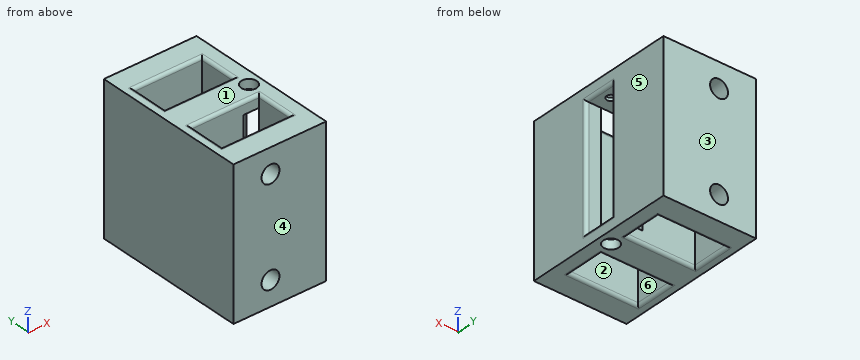
Autodesk Inventor part; units mm, degrees
ref_plane "YZ Plane" through (0, 0, 0) normal (1, 0, 0) x (0, 1, 0)
ref_plane "XZ Plane" through (0, 0, 0) normal (0, 1, 0) x (-1, 0, 0)
ref_plane "XY Plane" through (0, 0, 0) normal (0, 0, 1) x (1, 0, 0)
sketch "スケッチ1" plane through (0, 0, 0) normal (0, 1, 0) x (-1, 0, 0)
  line L0 (0, 0) -> (-30, 0)
  line L1 (-30, 0) -> (-30, -47.5)
  line L2 (-30, -47.5) -> (0, -47.5)
  line L3 (0, -47.5) -> (0, 0)
  dimension "d0" = 30
  dimension "d1" = 47.5
extrude "押し出し1" add sketch "スケッチ1" along normal blind 50
ref_plane "作業平面1" through (30, 0, 0) normal (1, 0, 0) x (0, 0, -1)
sketch "スケッチ2" plane through (30, 0, 0) normal (1, 0, 0) x (0, 0, -1)
  line L0 (4, 30) -> (43.5, 30)
  line L1 (43.5, 30) -> (43.5, 20)
  line L2 (43.5, 20) -> (4, 20)
  line L3 (4, 20) -> (4, 30)
  line L4 (0, 0) -> (0, 50)
  line L5 (0, 0) -> (0, 50)
  line L6 (0, 50) -> (47.5, 50)
  point P0 (0, 25)
  point P1 (4, 25)
  point P2 (0, 25)
  point P3 (23.75, 30)
  point P4 (23.75, 50)
  point P5 (23.75, 50)
  dimension "d5" = 39.5
  dimension "d6" = 10
  dimension "d7" = 0
  dimension "d8" = 0
extrude "押し出し2" cut sketch "スケッチ2" against normal blind 10
sketch "スケッチ3" plane through (0, 0, 0) normal (0, 0, 1) x (1, 0, 0)
  line L0 (3, 42) -> (25, 42)
  line L1 (25, 42) -> (25, 30)
  line L2 (25, 30) -> (3, 30)
  line L3 (3, 30) -> (3, 42)
  line L4 (0, 50) -> (30, 50)
  line L5 (3, 20) -> (25, 20)
  line L6 (25, 20) -> (25, 8)
  line L7 (25, 8) -> (3, 8)
  line L8 (3, 8) -> (3, 20)
  line L9 (0, 0) -> (30, 0)
  line L10 (0, 0) -> (0, 50)
  point P0 (14, 42)
  point P1 (15, 50)
  point P2 (15, 50)
  point P3 (14, 8)
  point P4 (15, 0)
  point P5 (15, 0)
  dimension "d11" = 22
  dimension "d12" = 12
  dimension "d13" = 8
  dimension "d14" = 22
  dimension "d15" = 12
  dimension "d16" = 8
  dimension "d48" = 3
  dimension "d49" = 3
extrude "押し出し3" cut sketch "スケッチ3" against normal through all
ref_plane "作業平面2" through (0, 50, 0) normal (0, 1, 0) x (1, 0, 0)
sketch "スケッチ4" plane through (0, 50, 0) normal (0, 1, 0) x (1, 0, 0)
  line L0 (30, 57) -> (30, -9.5)
  line L1 (30, 47.5) -> (0, 47.5)
  line L2 (0, 0) -> (30, 0)
  line L3 (0, 47.5) -> (0, 0)
  point P0 (12, 39.5)
  point P1 (12, 8)
  dimension "d24" = 8
  dimension "d25" = 8
  dimension "d52" = 12
  dimension "d53" = 12
hole "穴1" at (12, 50, -39.5) at (12, 50, -8) direction (0, -1, 0) diameter 5.8 depth 7
sketch "スケッチ5" plane through (0, 0, 0) normal (0, 0, 1) x (1, 0, 0)
  line L0 (30, 0) -> (30, 50)
  circle A0 centre (26, 25) radius 1.5
  point P0 (0, 0)
  point P1 (30, 25)
  point P2 (30, 25)
  dimension "d33" = 4
  dimension "d34" = 3
hole "穴2" at (26, 25, 0) direction (0, 0, -1) diameter 2.85 end through all
sketch "スケッチ6" plane through (0, 0, 0) normal (0, 0, 1) x (1, 0, 0)
  circle A0 centre (26, 25) radius 1.425
  circle A1 centre (26, 25) radius 2.5
  point P0 (0, 0)
  dimension "d42" = 5
extrude "押し出し4" cut sketch "スケッチ6" against normal blind 3 contours A0 | A1
sketch "スケッチ7" plane through (30, 0, -47.5) normal (0, 0, -1) x (-1, 0, 0)
  circle A0 centre (4, 25) radius 1.425
  circle A1 centre (4, 25) radius 2.5
  point P0 (30, 0)
  dimension "d45" = 5
extrude "押し出し5" cut sketch "スケッチ7" against normal blind 3 contours A0 | A1
fillet "フィレット1" radius 1 4 edges at (30, 25, -43.5) (30, 30, -23.75) (30, 20, -23.75) (30, 25, -4)
fillet "フィレット2" radius 1 16 edges at (3, 36, 0) (14, 42, 0) (14, 30, 0) (25, 36, 0) (25, 14, 0) (14, 20, 0) (3, 14, 0) (14, 8, 0) (3, 36, -47.5) (14, 42, -47.5) (25, 36, -47.5) (14, 30, -47.5) (14, 20, -47.5) (3, 14, -47.5) (25, 14, -47.5) (14, 8, -47.5)
ref_plane "作業平面3" through (0, 0, 0) normal (0, -1, 0) x (1, 0, 0)
sketch "スケッチ8" plane through (0, 0, 0) normal (0, -1, 0) x (1, 0, 0)
  circle A0 centre (12, -8) radius 2.9
  circle A1 centre (12, -39.5) radius 2.9
  point P0 (0, 0)
hole "穴3" at (12, 0, -8) at (12, 0, -39.5) direction (0, 1, 0) diameter 5.8 depth 7
properties part number "motor_rot_born1_3D プリント"
Read the model definition and answer for the solid it produces. Units are mm, in the model's axes. Face numbers are marked on the shaded views. A direction names the side the tool comes from. Round coordinates to 2 decimals unless told otherwise and drop trailing zeros. Write each loop counter-clockwise with the first axis right and the second up, starting at its lowest first coordinate (ties: lowest second). Pieces come first, ordered by that corner, then holes. Notation, with made-up numbers: (2, 24.25) - (49, 24.25) arc R20 cw to (49, 28.25) - close; hole circle Ø9 at (44.25, 21.25). An arc over 180 degrees is marked (long way). One line per item, written item: value.
Q1. Find section C-C (y = 25). Determine the outline of the cut face in (x, z) (3 decimals), and give its area (3 significant figures).
The answers:
outline: (0, -47.5) - (23.5, -47.5) - (23.5, -44.5) - (24.575, -44.5) - (24.575, -43.5) - (20, -43.5) - (20, -4) - (24.575, -4) - (24.575, -3) - (23.5, -3) - (23.5, 0) - (0, 0) - close; (27.425, -44.5) - (28.5, -44.5) - (28.5, -47.5) - (30, -47.5) - (30, -44.5) arc R1 ccw to (29, -43.5) - (27.425, -43.5) - close; (27.425, -4) - (29, -4) arc R1 ccw to (30, -3) - (30, 0) - (28.5, 0) - (28.5, -3) - (27.425, -3) - close
area: 994 mm2
Q2. Which of the six approach directions +Z, -Z, +X, -X, +Y, -Y give full straight-line access (tool end or side, diameter ignored) to the marked faces 1 and 2?
The answers:
face 1: +Z, +X, -X, +Y, -Y
face 2: +Z, -Z
Q3. For a pull along Y with two mould halves and no side action, classify the marked faces 3, 4, 5 and 6 as pulls with the +Y half, pulls with the -Y half, needs draft (parallel to the pull), parting line crosses it, or undercut.
The answers:
face 3: pulls with the +Y half
face 4: pulls with the -Y half
face 5: needs draft
face 6: undercut
Q4. Straight lines are drawn through the part: line 1 (Y direction, x = 18.5, z = -34); line 2 (Z direction, x = 12, y = 46.75); line 3 (Y direction, x = 26, z = -1.35). For each, find the intervals that lie inside material, in ascending order. Write a range as from..to.
The answers:
line 1: y = 0..8, 20..30, 42..50
line 2: z = -47.5..-42.4, -36.6..-10.9, -5.1..0
line 3: y = 0..22.5, 27.5..50
Q5. Each of these flat-tipped pins is pushed along its axis until it touches: P1, Ø1.5, axis at x = 26.5, y = 25.5, coming from the -Z side; P2, Ø1.5, axis at x = 27, y = 25, coming from the +Z side; P3, Ø3, axis at x = 13, z = -8.5, coming from the -Y side; P4, Ø2.5, axis at x = 26, y = 25, coming from the -Z side. Where does it stop, or does it pass through?
The answers:
P1: stops at z = -44.5
P2: stops at z = -3
P3: stops at y = 7
P4: passes through
Q6. Find section D-D (z = -26.5). Determine the outline of the cut face in (x, y).
The answers:
outline: (0, 0) - (30, 0) - (30, 19) arc R1 ccw to (29, 20) - (25, 20) - (25, 8) - (3, 8) - (3, 20) - (20, 20) - (20, 30) - (3, 30) - (3, 42) - (25, 42) - (25, 30) - (29, 30) arc R1 ccw to (30, 31) - (30, 50) - (0, 50) - close
Q7. Find section A-A (y = 11). Determine the outline of the cut face in (x, z), and give its area (3 significant figures).
The answers:
outline: (0, -47.5) - (2, -47.5) arc R1 ccw to (3, -46.5) - (3, -1) arc R1 ccw to (2, 0) - (0, 0) - close; (25, -46.5) arc R1 ccw to (26, -47.5) - (30, -47.5) - (30, 0) - (26, 0) arc R1 ccw to (25, -1) - close
area: 379 mm2
Q8. Find section B-B (x = 7.75). Determine the outline of the cut face in (y, z), and give its area (3 significant figures).
The answers:
outline: (0, -47.5) - (7, -47.5) arc R1 ccw to (8, -46.5) - (8, -1) arc R1 ccw to (7, 0) - (0, 0) - close; (20, -46.5) arc R1 ccw to (21, -47.5) - (29, -47.5) arc R1 ccw to (30, -46.5) - (30, -1) arc R1 ccw to (29, 0) - (21, 0) arc R1 ccw to (20, -1) - close; (42, -46.5) arc R1 ccw to (43, -47.5) - (50, -47.5) - (50, 0) - (43, 0) arc R1 ccw to (42, -1) - close
area: 1,230 mm2
